The listing builds one solid part. Answer for the finished solid, in the listing's coordinates (mm). Face numbers are marked on the shaded views. A direction names the side the tool comes from. Round coordinates to 2 decimals unless told otherwise and drop trailing zeros. Write each loop counter-clockwise with the first axis right and the second up, starting at its lowest first coordinate (ties: lowest second). Pieces come first, ordered by that corner, then holes. Notation, with made-up numbers: (30.25, 69.25) - (46.25, 69.25) arc R28 ccw to (46.25, 107.25) - close; hole circle Ø6 at (-29.5, -19.75). An arc over 180 degrees is marked (long way). Use a Markdown table: item, result. Add a question column.
1) A tool of negligible diameter and unlimited length cuts with its end or side. For the marked faces 4, 5 and 6, from which of +Z, -Z, +X, -X, +Y, -Y can it reach the whole face along a straight path? Write none if from no direction.
2) A cutting plane is placed at A-A (x = 11.5). Give the vertices of the cut face in (y, z).
3) Find the intervals of material crossed by probe 1 along X at (y, z) = (7.5, 6); probe 2 along Z at (x, y) = (12, 7.5); probe 3 along X at (y, z) = (11, -7), in increasing order. Write a range as from..to.
4) This flat-tipped pin is pushed along its axis until it touches: P1, Ø5, axis at x = 8, y = 18, coming from the -Z side (3 decimals). Where does it stop, or does it pass through?
5) Determine the mould class of the marked faces 1, 2 and 3 for opening direction Z: +Z half, -Z half, draft (parallel to the pull), parting line (faces both ways), or undercut.
```python
from build123d import *

# Parameters (mm, degrees)
SKETCH1_R           = 18.05
BOSS_EXTRUDE1_DEPTH = 21.5
SKETCH2_R           = 1
CUT_EXTRUDE1_DEPTH  = 34.374466288
CUT_EXTRUDE2_DEPTH  = 34.374466288
CIRPATTERN1_COUNT   = 20


with BuildPart() as part:
    # Sketch1 → Boss-Extrude1 (new body)
    with BuildSketch(Plane(origin=(0, 0, 0), x_dir=(1, 0, 0), z_dir=(0, 1, 0))):
        with Locations(Location((0, 0, 0), (0, 0, 270))):
            Circle(SKETCH1_R)
    extrude(amount=BOSS_EXTRUDE1_DEPTH)

    # Sketch2 → Cut-Extrude1 (cut, through all)
    with BuildSketch(Plane(origin=(0, 21.5, 0), x_dir=(1, 0, 0), z_dir=(0, 1, 0))):
        with Locations(Location((-9.25, 0, 0), (0, 0, 270))):
            Circle(SKETCH2_R)
        with Locations(Location((0, 9.25, 0), (0, 0, 270))):
            Circle(SKETCH2_R)
        with Locations(Location((9.25, 0, 0), (0, 0, 270))):
            Circle(SKETCH2_R)
        with Locations(Location((0, -9.25, 0), (0, 0, 270))):
            Circle(SKETCH2_R)
    extrude(amount=-CUT_EXTRUDE1_DEPTH, mode=Mode.SUBTRACT)

    # Sketch3 → Cut-Extrude2 (cut, through all)
    with BuildSketch(Plane(origin=(0, 21.5, 0), x_dir=(1, 0, 0), z_dir=(0, 1, 0))):
        with BuildLine():
            ThreePointArc((2.161718459, 17.92008575), (0, 18.05), (-2.161718459, 17.92008575))
            Line((-2.161718459, 17.92008575), (-0.502594701, 10.114522161))
            ThreePointArc((-0.502594701, 10.114522161), (0, 10.25), (0.502594701, 10.114522161))
            Line((0.502594701, 10.114522161), (2.161718459, 17.92008575))
        make_face()
        with BuildLine():
            ThreePointArc((0.502594701, 10.114522161), (0, 10.25), (-0.502594701, 10.114522161))
            Line((-0.502594701, 10.114522161), (-0.107510264, 8.255796025))
            ThreePointArc((-0.107510264, 8.255796025), (0, 8.25), (0.107510264, 8.255796025))
            Line((0.107510264, 8.255796025), (0.502594701, 10.114522161))
        make_face()
        with BuildLine():
            ThreePointArc((0.107510264, 8.255796025), (0, 8.25), (-0.107510264, 8.255796025))
            Line((-0.107510264, 8.255796025), (0, 7.75))
            Line((0, 7.75), (0.107510264, 8.255796025))
        make_face()
    cut_extrude2 = extrude(amount=-CUT_EXTRUDE2_DEPTH, mode=Mode.SUBTRACT)

    # CirPattern1: Cut-Extrude2 ×20 about axis
    cirpattern1_axis = Axis((0, 0, 0), (0, 1, 0))
    for i in range(1, CIRPATTERN1_COUNT):
        add(cut_extrude2.rotate(cirpattern1_axis, i * 360 / CIRPATTERN1_COUNT), mode=Mode.SUBTRACT)


solid = part.part
```
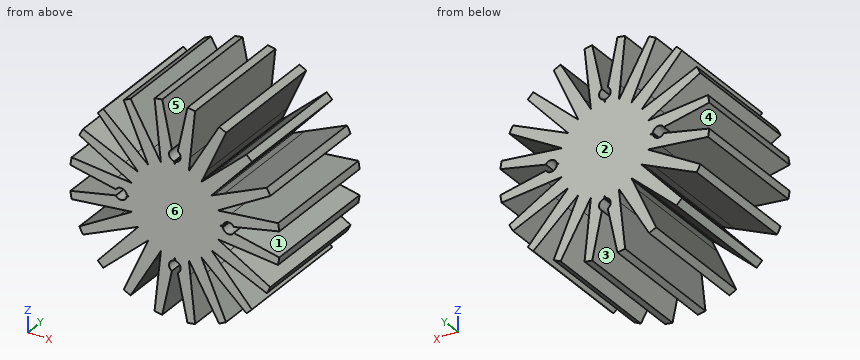
Entries:
| question | item | result |
|---|---|---|
| 1 | face 4 | -X, +Y, -Y |
| 1 | face 5 | +Z, +Y, -Y |
| 1 | face 6 | +Z, -Z, +X, -X, -Y |
| 2 | outline | (0, -12.52) - (21.5, -12.52) - (21.5, -10.36) - (0, -10.36) - close; (0, -6.88) - (21.5, -6.88) - (21.5, -4.78) - (0, -4.78) - close; (0, -2.83) - (21.5, -2.83) - (21.5, -0.8) - (0, -0.8) - close; (0, 0.8) - (21.5, 0.8) - (21.5, 2.83) - (0, 2.83) - close; (0, 4.78) - (21.5, 4.78) - (21.5, 6.88) - (0, 6.88) - close; (0, 10.36) - (21.5, 10.36) - (21.5, 12.52) - (0, 12.52) - close |
| 3 | probe 1 | x = -13.61..-9.51, -7.57..7.57, 9.51..13.61 |
| 3 | probe 2 | z = -12.97..-10.92, -7.11..-5.07, -2.88..-0.9, 0.9..2.88, 5.07..7.11, 10.92..12.97 |
| 3 | probe 3 | x = -15.35..-11.76, -8.47..-5.37, -4.88..4.88, 5.37..8.47, 11.76..15.35 |
| 4 | P1 | stops at z = -16.375 |
| 5 | face 1 | undercut |
| 5 | face 2 | draft |
| 5 | face 3 | -Z half |
